Part model, mm, in its own coordinate system. A direction names the side the tool comes from. Coordinates: 2 decimals unless noted, no trailing zeros. Order: outer loops, then holes, each group sorted by start corner. A loop starts at its lowest first (then second) coordinate and runs counter-clockwise, first axis right, second up.
1) Cut at A-A (y = 108.5). List the corners of the cut face in (x, z), and give its area (3 significant figures).
2) Mould opens along X. For faces 4 (the flat face through (37.31, 83.92, 46.56)), 5 (the flat face through (45, 90, 38.1)), 6 (the flat face through (0, 67, 3)) say: +X half, -X half, draft (parallel to the pull), parting line (faces both ways), or undercut.
3) Cut at D-D (x = 191.5). List the corners of the cut face in (y, z), and give its area (3 significant figures).
4) Tool access for faces 1 (the flat face through (44, 93.491, 44)), 2 (the flat face through (63.5, 84, 29)), 3 (the flat face through (25.4, 84, 29)): list every direction of +Z, -Z, +X, -X, +Y, -Y with a clear straight run to the whole face (end or side of a thin tool).
5) Cut at B-B (z = 28). List the corners of the cut face in (x, y).
6) Cut at C-C (z = 46.5). List the corners of the cut face in (x, y).
7) Wall check: L1, parallel to Z at x = 26.5, y = 90; L2, parallel to X at y = 110, z = 26.5; L3, parallel to X at y = 85.5, z = 16. Give the ranges that are in metal, low to high.
8) Pin check, flat tips, straight feed: pin 1 Ø2 at (x, y) = (73, 45) entering from +Z; pin 2 Ø3 at (x, z) = (43, 36) entering from +Y; pin 3 Ø19 at (x, z) = (36, 33) entering from -Y; pin 4 Ø1.5 at (y, z) = (40.5, 8.5) entering from +X. Stop position of each tip, or through.
```python
from build123d import *

# Parameters (mm, degrees)
F0_W       = 355.6
F0_H       = 127
F1_DEPTH   = 6.35
F2_W       = 38.1
F2_H       = 6.35
F3_DEPTH   = 50.8
F3_FACE1_W = 38.1
F3_FACE1_H = 50.8
F5_DEPTH   = 50.8
F6_W       = 9.525
F6_H       = 25.4
F7_DEPTH   = 25.4
F8_W       = 9.525
F8_H       = 19.05
F9_DEPTH   = 12.7


with BuildPart() as f1:
    # F0 (on Top) → F1 (new body)
    with BuildSketch(Plane.XY):
        with Locations((177.8, 68.0911967754)):
            Rectangle(F0_W, F0_H)
    extrude(amount=F1_DEPTH)

    # F2 (on face) → F3 (join)
    with BuildSketch(Plane.XY.offset(6.35)):
        with Locations((44.45, 52.2161967754)):
            Rectangle(F2_W, F2_H)
        with Locations((44.45, 83.9661967754)):
            Rectangle(F2_W, F2_H)
    extrude(amount=F3_DEPTH)

    # F4 (on face) + F3_face1 (on face) → F5 (cut)
    with BuildSketch(Plane.XZ.offset(-49.0411967754)):
        Polygon((63.5, 57.15), (25.4, 57.15), (25.4, 52.3875), (30.3680338836, 52.3875), (44.45, 40.5713274255), (58.5319661164, 52.3875), (63.5, 52.3875), align=None)
    with BuildSketch(Plane(origin=(44.45, 87.1411967754, 31.75), x_dir=(-1, 0, 0), z_dir=(0, 1, 0))):
        Rectangle(F3_FACE1_W, F3_FACE1_H)
    extrude(amount=-F5_DEPTH, dir=(0, -1, 0), mode=Mode.SUBTRACT)

    # F6 (on face) → F7 (join)
    with BuildSketch(Plane(origin=(0, 87.1411967754, 0), x_dir=(-1, 0, 0), z_dir=(0, 1, 0))):
        with Locations((-44.45, 25.4)):
            Rectangle(F6_W, F6_H)
    extrude(amount=F7_DEPTH)

    # F8 (on face) → F9 (join)
    with BuildSketch(Plane.XY.offset(38.1)):
        with Locations((44.45, 103.0161967754)):
            Rectangle(F8_W, F8_H)
    extrude(amount=F9_DEPTH)


solid = f1.part
```
Geometry check:
1. outline: (0, 0) - (355.6, 0) - (355.6, 6.35) - (0, 6.35) - close; (39.69, 12.7) - (49.21, 12.7) - (49.21, 50.8) - (39.69, 50.8) - close
1. area: 2,620 mm2
2. face 4: undercut
2. face 5: draft
2. face 6: -X half
3. outline: (4.59, 0) - (131.59, 0) - (131.59, 6.35) - (4.59, 6.35) - close
3. area: 806 mm2
4. face 1: +Z, +X, -X
4. face 2: +Z, +X, +Y, -Y
4. face 3: +Z, -X, +Y, -Y
5. outline: (25.4, 49.04) - (63.5, 49.04) - (63.5, 55.39) - (25.4, 55.39) - close; (25.4, 80.79) - (63.5, 80.79) - (63.5, 87.14) - (49.21, 87.14) - (49.21, 112.54) - (39.69, 112.54) - (39.69, 87.14) - (25.4, 87.14) - close
6. outline: (25.4, 49.04) - (37.38, 49.04) - (37.38, 55.39) - (25.4, 55.39) - close; (25.4, 80.79) - (37.38, 80.79) - (37.38, 87.14) - (25.4, 87.14) - close; (39.69, 93.49) - (49.21, 93.49) - (49.21, 112.54) - (39.69, 112.54) - close; (51.52, 49.04) - (63.5, 49.04) - (63.5, 55.39) - (51.52, 55.39) - close; (51.52, 80.79) - (63.5, 80.79) - (63.5, 87.14) - (51.52, 87.14) - close
7. L1: z = 0 to 6.35
7. L2: x = 39.69 to 49.21
7. L3: x = 25.4 to 63.5
8. pin 1: stops at z = 6.35
8. pin 2: stops at y = 112.54
8. pin 3: stops at y = 49.04
8. pin 4: passes through
